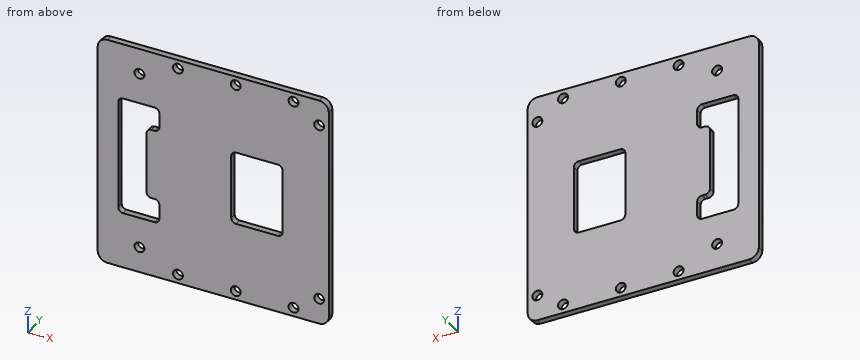
```python
from build123d import *

# Parameters (mm, degrees)
SKETCH1_W           = 72
SKETCH1_H           = 72
SKETCH1_R           = 1.55
SKETCH1_W_2         = 16
SKETCH1_H_2         = 23
BOSS_EXTRUDE1_DEPTH = 2
FILLET1_R           = 1.5
SKETCH2_W           = 4
SKETCH2_H           = 22
BOSS_EXTRUDE2_DEPTH = 2
FILLET3_R           = 1.5
FILLET5_R           = 3


with BuildPart() as part:
    # Sketch1 → Boss-Extrude1 (new body)
    with BuildSketch(Plane(origin=(0, 0, 0), x_dir=(1, 0, 0), z_dir=(0, 1, 0))):
        with Locations((-5.976585554, 0)):
            Rectangle(SKETCH1_W, SKETCH1_H)
        with Locations((-28.976585554, -28)):
            Circle(SKETCH1_R, mode=Mode.SUBTRACT)
        with Locations((-16.976585554, -33.25)):
            Circle(SKETCH1_R, mode=Mode.SUBTRACT)
        Polygon((-22.776585554, 18.5), (-22.776585554, -18.5), (-27, -18.5), (-35.576585554, -18.5), (-35.576585554, 18.5), (-31.976585554, 18.5), align=None, mode=Mode.SUBTRACT)
        with Locations((1.023414446, -33.25)):
            Circle(SKETCH1_R, mode=Mode.SUBTRACT)
        with Locations((19.023414446, -33.25)):
            Circle(SKETCH1_R, mode=Mode.SUBTRACT)
        with Locations((27.023414446, -28)):
            Circle(SKETCH1_R, mode=Mode.SUBTRACT)
        with Locations((-28.976585554, 28)):
            Circle(SKETCH1_R, mode=Mode.SUBTRACT)
        with Locations((-16.976585554, 33.25)):
            Circle(SKETCH1_R, mode=Mode.SUBTRACT)
        with Locations((7.623414446, 0)):
            Rectangle(SKETCH1_W_2, SKETCH1_H_2, mode=Mode.SUBTRACT)
        with Locations((1.023414446, 33.25)):
            Circle(SKETCH1_R, mode=Mode.SUBTRACT)
        with Locations((19.023414446, 33.25)):
            Circle(SKETCH1_R, mode=Mode.SUBTRACT)
        with Locations((27.023414446, 28)):
            Circle(SKETCH1_R, mode=Mode.SUBTRACT)
    extrude(amount=BOSS_EXTRUDE1_DEPTH)

    # Fillet1
    fillet1_edges = [part.edges().sort_by_distance(p)[0] for p in [
        (-0.376585554, 1, 11.5),
        (15.623414446, 1, 11.5),
        (15.623414446, 1, -11.5),
        (-0.376585554, 1, -11.5),
        (-35.576585554, 1, 18.5),
        (-22.776585554, 1, 18.5),
        (-22.776585554, 1, -18.5),
        (-35.576585554, 1, -18.5),
    ]]
    fillet(fillet1_edges, radius=FILLET1_R)

    # Sketch2 → Boss-Extrude2 (add)
    with BuildSketch(Plane(origin=(0, 2, 0), x_dir=(1, 0, 0), z_dir=(0, 1, 0))):
        with Locations((-24.776585554, 0)):
            Rectangle(SKETCH2_W, SKETCH2_H)
    extrude(amount=-BOSS_EXTRUDE2_DEPTH)

    # Fillet3
    fillet3_edges = [part.edges().sort_by_distance(p)[0] for p in [
        (-26.776585554, 1, 11),
        (-26.776585554, 1, -11),
        (-22.776585554, 1, -11),
        (-22.776585554, 1, 11),
    ]]
    fillet(fillet3_edges, radius=FILLET3_R)

    # Fillet5
    fillet5_edges = [part.edges().sort_by_distance(p)[0] for p in [
        (-41.976585554, 1, -36),
        (30.023414446, 1, -36),
        (30.023414446, 1, 36),
        (-41.976585554, 1, 36),
    ]]
    fillet(fillet5_edges, radius=FILLET5_R)


solid = part.part
```
The model under review builds one solid part; all positions refer to its coordinate system, in mm. Round coordinates to 2 decimals unless told otherwise and drop trailing zeros. Order: outer loops, then holes, each group sorted by start corner. A loop starts at its lowest first (then second) coordinate and runs counter-clockwise, first axis right, second up. Notation, with made-up numbers: M 75,39.5 L 114,39.5 A38 cw 114,78.5 Z; hole C -4.5,-2.5 d2. An arc over 180 degrees is marked long. Use a Markdown table: item, result.
1) Consider section A-A (x = -31.5). Write out the cut boundary in (y, z), then the cut area to 3 significant figures.
Report:
| item | result |
|---|---|
| outline | M 0,-36 L 2,-36 L 2,-18.5 L 0,-18.5 Z; M 0,18.5 L 2,18.5 L 2,36 L 0,36 Z |
| area | 70.0 mm^2 |
2) Consider section B-B (z = -8). Write out the cut boundary in (x, y).
Report:
| item | result |
|---|---|
| outline | M -41.98,0 L -35.58,0 L -35.58,2 L -41.98,2 Z; M -26.78,0 L -0.38,0 L -0.38,2 L -26.78,2 Z; M 15.62,0 L 30.02,0 L 30.02,2 L 15.62,2 Z |
3) Wall thickness on line 1 along X through (y, z) = (1.45, 28); line 2 along X through (y, z) = (0.45, 7); line 3 along Z through (x, y) = (-29, 1): over which ranges is each line inside the solid? List them lowest first. Write a range as [from, to].
Report:
| item | result |
|---|---|
| line 1 | [-41.98, -30.53], [-27.43, 25.47], [28.57, 30.02] |
| line 2 | [-41.98, -35.58], [-26.78, -0.38], [15.62, 30.02] |
| line 3 | [-36, -29.55], [-26.45, -18.5], [18.5, 26.45], [29.55, 36] |
4) Consider section D-D (y = 1.1). Give the number of separate pieces and of enclosed holes in the cut face, then the cut area to 3 significant figures.
Report:
| item | result |
|---|---|
| separate pieces | 1 |
| enclosed holes | 12 |
| area | 4,350 mm^2 |
5) Consider section C-C (x = -17). Write out the cut boundary in (y, z).
Report:
| item | result |
|---|---|
| outline | M 0,-36 L 2,-36 L 2,-34.8 L 0,-34.8 Z; M 0,-31.7 L 2,-31.7 L 2,31.7 L 0,31.7 Z; M 0,34.8 L 2,34.8 L 2,36 L 0,36 Z |
